from build123d import *

# Parameters (mm, degrees)
SKETCH_1_R          = 10
SKETCH_1_R_2        = 5
EXTRUDE_1_DEPTH     = 10
SKETCH_2_R          = 10
SKETCH_2_R_2        = 4
EXTRUDE_2_DEPTH     = 10
CUT_EXTRUDE_START   = -10
CUT_EXTRUDE_1_DEPTH = 10
SKETCH_4_R          = 7
CUT_EXTRUDE_2_DEPTH = 10


with BuildPart() as part:
    # 草图1 → 凸台-拉伸1 (new body)
    with BuildSketch(Plane.XY):
        Circle(SKETCH_1_R)
        Circle(SKETCH_1_R_2, mode=Mode.SUBTRACT)
    extrude(amount=EXTRUDE_1_DEPTH)

    # 草图2 → 凸台-拉伸2 (add)
    with BuildSketch(Plane.XY.offset(10)):
        Circle(SKETCH_2_R)
        Circle(SKETCH_2_R_2, mode=Mode.SUBTRACT)
    extrude(amount=EXTRUDE_2_DEPTH)

    # 草图3 → 切除-拉伸1 (cut)
    with BuildSketch(Plane.XY.offset(20).offset(CUT_EXTRUDE_START)):
        with BuildLine():
            Line((2.678784027, 6.467156728), (3.826834324, 9.238795325))
            ThreePointArc((3.826834324, 9.238795325), (0, 10), (-3.826834324, 9.238795325))
            Line((-3.826834324, 9.238795325), (-2.678784027, 6.467156728))
            ThreePointArc((-2.678784027, 6.467156728), (0, 7), (2.678784027, 6.467156728))
        make_face()
        with BuildLine():
            ThreePointArc((10, 0), (9.807852804, 1.95090322), (9.238795325, 3.826834324))
            Line((9.238795325, 3.826834324), (6.467156728, 2.678784027))
            ThreePointArc((6.467156728, 2.678784027), (7, 0), (6.467156728, -2.678784027))
            Line((6.467156728, -2.678784027), (9.238795325, -3.826834324))
            ThreePointArc((9.238795325, -3.826834324), (9.807852804, -1.95090322), (10, 0))
        make_face()
        with BuildLine():
            Line((-2.678784027, -6.467156728), (-3.826834324, -9.238795325))
            ThreePointArc((-3.826834324, -9.238795325), (0, -10), (3.826834324, -9.238795325))
            Line((3.826834324, -9.238795325), (2.678784027, -6.467156728))
            ThreePointArc((2.678784027, -6.467156728), (0, -7), (-2.678784027, -6.467156728))
        make_face()
        with BuildLine():
            Line((-6.467156728, 2.678784027), (-9.238795325, 3.826834324))
            ThreePointArc((-9.238795325, 3.826834324), (-10, 0), (-9.238795325, -3.826834324))
            Line((-9.238795325, -3.826834324), (-6.467156728, -2.678784027))
            ThreePointArc((-6.467156728, -2.678784027), (-7, 0), (-6.467156728, 2.678784027))
        make_face()
    extrude(amount=CUT_EXTRUDE_1_DEPTH, mode=Mode.SUBTRACT)

    # 草图4 → 切除-拉伸2 (cut)
    with BuildSketch(Plane.XY.offset(20).offset(CUT_EXTRUDE_START)):
        Circle(SKETCH_4_R)
    extrude(amount=CUT_EXTRUDE_2_DEPTH, mode=Mode.SUBTRACT)


solid = part.part
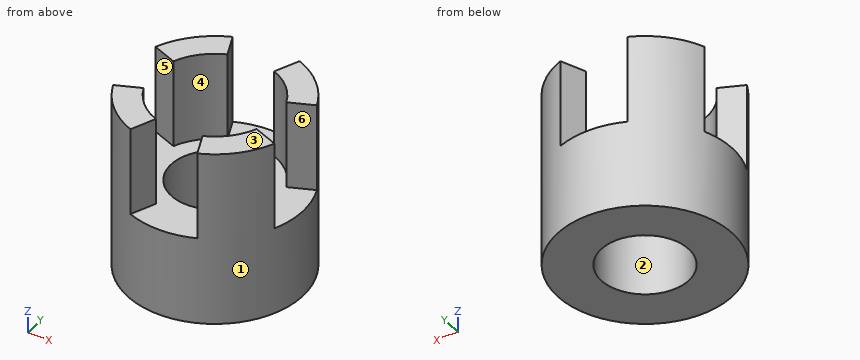
CAD build for the part. Positions are in the model's coordinates, mm. Face numbers are marked on the shaded views. A direction names the side the tool comes from. Round coordinates to 2 decimals unless told otherwise and drop trailing zeros. Loops run counter-clockwise (first coordinate to the right, second up) from the corner with the lowest first, then second, coordinate; pieces in that order, holes last. Notation, with made-up numbers: M 67,58.25 L 85,58.25 A9 ccw 85,75.25 Z; hole C 9,-9.5 d8. An arc over 180 degrees is marked long. One line per question, with ' | ' between items. Start each with the question number.
Item 1: Cut at D-D, the plane z = 2.25. Write the cut outline in (x, y), plus the area to 3 significant figures.
Item 2: Pin check, flat tips, straight feed: pin 1 Ø1.5 at (x, z) = (-2, 5) entering from +Y; pin 2 Ø5 at (x, y) = (0, -4) entering from +Z; pin 3 Ø10 at (y, z) = (3, 17.5) entering from -X. Stop position of each tip, or through.
Item 3: Cut at C-C, the plane z = 11. Write the cut outline in (x, y), plus the area to 3 significant figures.
Item 4: Which spindle directions (+Z, -Z, +X, -X, +Y, -Y) get a long thin tool onto all of the face, cutting with end or side? Do the marked faces 4, 5 and 6. Say none if no direction does.
Item 5: Cut at A-A, the plane x = 0. Write the cut outline in (y, z), plus the area to 3 significant figures.
Item 6: Wall check: line 1 (Y direction, x = 0, z = 7.25); line 2 (Y direction, x = -8.75, z = 15.75); line 3 (Z direction, x = -2.75, y = -4.5). Give the ranges that are in metal, low to high.
Item 7: Two-plate mould, pull along X, no slides. Class the marked faces 1, 2 and 3: pulls with the +X half, pulls with the -X half, needs draft (parallel to the pull), parting line crosses it, or undercut.
Responses:
1) outline: C 0,0 d20; hole C 0,0 d10 | area: 236 mm²
2) pin 1: stops at y = 9.92 | pin 2: stops at z = 10 | pin 3: stops at x = -9.24
3) outline: M -9.24,-3.83 A10 ccw -3.83,-9.24 L -2.68,-6.47 A7 cw -6.47,-2.68 Z; M -9.24,3.83 L -6.47,2.68 A7 cw -2.68,6.47 L -3.83,9.24 A10 ccw Z; M 2.68,-6.47 L 3.83,-9.24 A10 ccw 9.24,-3.83 L 6.47,-2.68 A7 cw Z; M 2.68,6.47 A7 cw 6.47,2.68 L 9.24,3.83 A10 ccw 3.83,9.24 Z | area: 80.1 mm²
4) face 4: +Z | face 5: +Z, -X | face 6: +Z, +X
5) outline: M -10,0 L -5,0 L -5,10 L -10,10 Z; M 5,0 L 10,0 L 10,10 L 5,10 Z | area: 100 mm²
6) line 1: y = -10 to -5, 5 to 10 | line 2: y = -4.84 to -3.62, 3.62 to 4.84 | line 3: z = 0 to 10
7) face 1: parting line crosses it | face 2: undercut | face 3: needs draft
